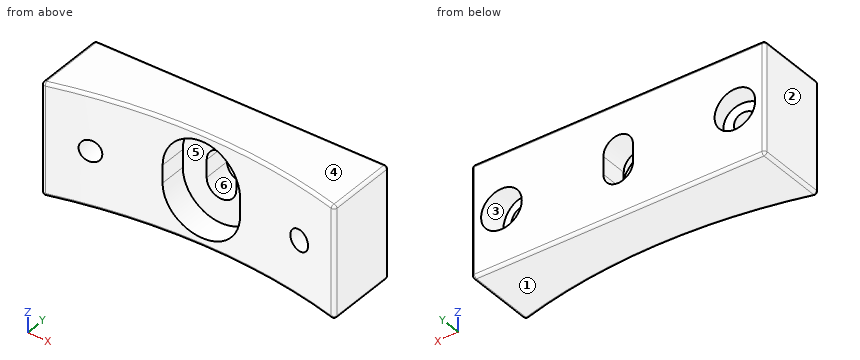
from build123d import *

# Parameters (mm, degrees)
BOSS_EXTRUDE1_DEPTH     = 24.13
FILLET1_R               = 0.635
CUT_EXTRUDE1_DEPTH      = 43.849527948
CUT_EXTRUDE6_DEPTH      = 42.512826607
CUT_EXTRUDE6_DEPTH_BACK = 5.588


with BuildPart() as part:
    # Sketch1 → Boss-Extrude1 (new body)
    with BuildSketch(Plane.XY):
        with BuildLine():
            Line((-31.75, 12.7), (31.75, 12.7))
            Line((31.75, 12.7), (31.75, -3.175))
            ThreePointArc((31.75, -3.175), (0, 1.167638116), (-31.75, -3.175))
            Line((-31.75, -3.175), (-31.75, 12.7))
        make_face()
    extrude(amount=BOSS_EXTRUDE1_DEPTH)

    # Sketch5 → Cut-Revolve1 (revolve, cut)
    with BuildSketch(Plane(origin=(0, 0, 12.065), x_dir=(-1, 0, 0), z_dir=(0, 0, -1)), mode=Mode.PRIVATE) as cut_revolve1_sk:
        Polygon((-22.482530384, -1.647401081), (-24.72635964, -2.084466602), (-26.680337626, 7.946965208), (-28.67485252, 7.558462523), (-30.361328492, 16.216578855), (-26.122984342, 17.042147061), align=None)
    cut_revolve1 = revolve(cut_revolve1_sk.sketch.rotate(Axis((26.472561187, 18.836822495, 12.065), (-0.19119226638023634, -0.9815526054554533, 0)), 180), axis=Axis((26.472561187, 18.836822495, 12.065), (-0.19119226638023634, -0.9815526054554533, 0)), mode=Mode.SUBTRACT)

    # Mirror1: Cut-Revolve1 across plane
    add(cut_revolve1.mirror(Plane(origin=(0, 0, 0), x_dir=(0, 0, 1), z_dir=(1, 0, 0))), mode=Mode.SUBTRACT)

    # Fillet1
    fillet1_edges = [part.edges().sort_by_distance(p)[0] for p in [
        (0, 12.7, 24.13),
        (-31.75, 4.7625, 24.13),
        (0, 1.167638116, 24.13),
        (-31.75, 4.7625, 0),
        (0, 12.7, 0),
        (31.75, 4.7625, 0),
        (0, 1.167638116, 0),
        (31.75, 4.7625, 24.13),
        (-31.75, -3.175, 12.065),
        (-31.75, 12.7, 12.065),
        (31.75, 12.7, 12.065),
        (31.75, -3.175, 12.065),
    ]]
    fillet(fillet1_edges, radius=FILLET1_R)

    # Sketch17 → Cut-Extrude1 (cut, through all)
    with BuildSketch(Plane(origin=(0, 12.7, 0), x_dir=(1, 0, 0), z_dir=(0, 1, 0))):
        with BuildLine():
            Line((-3.2004, -13.97), (-3.2004, -10.16))
            ThreePointArc((-3.2004, -10.16), (0, -6.9596), (3.2004, -10.16))
            Line((3.2004, -10.16), (3.2004, -13.97))
            ThreePointArc((3.2004, -13.97), (0, -17.1704), (-3.2004, -13.97))
        make_face()
    extrude(amount=-CUT_EXTRUDE1_DEPTH, mode=Mode.SUBTRACT)

    # Sketch18 → Cut-Extrude6 (cut, two sides: drawn at the far end of the back side and taken through both)
    with BuildSketch(Plane(origin=(0, 1.167638116, 0), x_dir=(-1, 0, 0), z_dir=(0, -1, 0)).offset(-CUT_EXTRUDE6_DEPTH_BACK)):
        with BuildLine():
            Line((8.382, -10.16), (8.382, -13.97))
            ThreePointArc((8.382, -13.97), (0, -22.352), (-8.382, -13.97))
            Line((-8.382, -13.97), (-8.382, -10.16))
            ThreePointArc((-8.382, -10.16), (0, -1.778), (8.382, -10.16))
        make_face()
    extrude(amount=CUT_EXTRUDE6_DEPTH + CUT_EXTRUDE6_DEPTH_BACK, mode=Mode.SUBTRACT)


solid = part.part
Work out the finished part from the listing and answer in its coordinate system (mm). Face numbers are marked on the shaded views. A direction names the side the tool comes from. Give positions to 0.01 mm unless a question says otherwise; leave off trailing zeros. Write each loop counter-clockwise with the first axis right and the second up, starting at its lowest first coordinate (ties: lowest second). Pieces come first, ordered by that corner, then holes. Notation, with made-up numbers: (-13.75, 0) - (2.25, 0) arc R12 cw to (2.25, 14) - close; hole circle Ø6 at (0, -17.75). An arc over 180 degrees is marked (long way). One line per item, written item: value. Start each with the question number.
1. For the marked faces 4, 5 and 6, determine the directions among +Z, -Z, +X, -X, +Y, -Y from which every point of the face is accessible in a straight line to the end or side of a thin tool.
2. Find section D-D (z = 19.75). Write down the section's boundary in (x, y) (3 decimals), then the cut area to 3 significant figures.
3. Find section A-A (x = 0). Write down the section's boundary in (y, z) (3 decimals).
4. Find section B-B (z = 5). Write down the section's boundary in (x, y) (3 decimals).
5. Find section C-C (y = 3.75). State how many separate pieces and enclosed holes the cut face has, then the cut area to 3 significant figures.
6. Given pin 1 (13.5 mm diameter, centred on x = 1, z = 9.5, fed in from -Y); pin 2 (1.5 mm diameter, centred on x = -12, z = 10, fed in from -Y); pin 3 (5 mm diameter, centred on x = -16.5, z = 11, fed in from -Y), each flat-ended and moving along its own axis, determine where each tip first touches the part or whether it passes through.
7. For a pull along Z with two mould halves and no side action, classify the marked faces 1, 2 and 3 as +Z half, -Z half, draft (parallel to the pull), parting line (faces both ways), or undercut.
8. Consider probe 1 along Z at (x, y) = (23.5, 2.5); probe 2 along X at (y, z) = (2.25, 12.25); probe 3 along X at (y, z) = (7, 14). Determine where each line is inside the solid, lowest interval first.
Geometry results:
1. face 4: +Z, +X, -X, +Y, -Y
1. face 5: -Y
1. face 6: +Y, -Y
2. outline: (-31.75, -2.342) arc R0.635 ccw to (-30.949, -2.955) arc R118.237 cw to (-6.07, 1.012) - (-6.07, 6.756) - (6.07, 6.756) - (6.07, 1.012) arc R118.237 cw to (30.949, -2.955) arc R0.635 ccw to (31.75, -2.342) - (31.75, 12.065) arc R0.635 ccw to (31.115, 12.7) - (-31.115, 12.7) arc R0.635 ccw to (-31.75, 12.065) - close
2. area: 755 mm2
3. outline: (1.168, 0.635) arc R0.635 ccw to (1.803, 0) - (12.065, 0) arc R0.635 ccw to (12.7, 0.635) - (12.7, 6.96) - (6.756, 6.96) - (6.756, 1.778) - (1.168, 1.778) - close; (1.168, 22.352) - (6.756, 22.352) - (6.756, 17.17) - (12.7, 17.17) - (12.7, 23.495) arc R0.635 ccw to (12.065, 24.13) - (1.803, 24.13) arc R0.635 ccw to (1.168, 23.495) - close
4. outline: (-31.75, -2.342) arc R0.635 ccw to (-30.949, -2.955) arc R118.237 cw to (-6.605, 0.983) - (-6.605, 6.756) - (6.605, 6.756) - (6.605, 0.983) arc R118.237 cw to (30.949, -2.955) arc R0.635 ccw to (31.75, -2.342) - (31.75, 12.065) arc R0.635 ccw to (31.115, 12.7) - (-31.115, 12.7) arc R0.635 ccw to (-31.75, 12.065) - close
5. separate pieces: 1
5. enclosed holes: 3
5. area: 1,210 mm2
6. pin 1: y = 6.76
6. pin 2: y = 0.48
6. pin 3: y = -0.37
7. face 1: -Z half
7. face 2: draft
7. face 3: undercut
8. probe 1: 0 to 9.79, 14.34 to 24.13
8. probe 2: -31.75 to -25.56, -20.92 to -8.38, 8.38 to 20.92, 25.56 to 31.75
8. probe 3: -31.75 to -25.41, -22.93 to -3.2, 3.2 to 22.93, 25.41 to 31.75
